from build123d import *

# Parameters (mm, degrees)
CROQUIS1_R              = 1.5
SALIENTE_EXTRUIR1_DEPTH = 1.6
CROQUIS2_W              = 40
CROQUIS2_H              = 3.2
SALIENTE_EXTRUIR2_DEPTH = 40


with BuildPart() as part:
    # Croquis1 → Saliente-Extruir1 (new, symmetric)
    with BuildSketch(Plane.XY):
        with BuildLine():
            Line((-20, -23.5), (20, -23.5))
            Line((20, -23.5), (20, 4.5))
            ThreePointArc((20, 4.5), (14.435028843, 17.935028843), (1, 23.5))
            Line((1, 23.5), (-1, 23.5))
            ThreePointArc((-1, 23.5), (-14.435028843, 17.935028843), (-20, 4.5))
            Line((-20, 4.5), (-20, -23.5))
        make_face()
        with Locations((-15.5, 0)):
            Circle(CROQUIS1_R, mode=Mode.SUBTRACT)
        with Locations((-7.75, 13.423393759)):
            Circle(CROQUIS1_R, mode=Mode.SUBTRACT)
        with Locations((7.75, 13.423393759)):
            Circle(CROQUIS1_R, mode=Mode.SUBTRACT)
        with Locations((15.5, 0)):
            Circle(CROQUIS1_R, mode=Mode.SUBTRACT)
        with Locations((7.75, -13.423393759)):
            Circle(CROQUIS1_R, mode=Mode.SUBTRACT)
        with Locations((-7.75, -13.423393759)):
            Circle(CROQUIS1_R, mode=Mode.SUBTRACT)
        with BuildLine():
            Line((6.5, 7.5), (6.5, -7.5))
            ThreePointArc((6.5, -7.5), (0, -14), (-6.5, -7.5))
            Line((-6.5, -7.5), (-6.5, 7.5))
            ThreePointArc((-6.5, 7.5), (0, 14), (6.5, 7.5))
        make_face(mode=Mode.SUBTRACT)
    extrude(amount=SALIENTE_EXTRUIR1_DEPTH, both=True)

    # Croquis2 → Saliente-Extruir2 (add)
    with BuildSketch(Plane(origin=(0, 0, -1.6), x_dir=(-1, 0, 0), z_dir=(0, 0, -1))):
        with Locations((0, -21.9)):
            Rectangle(CROQUIS2_W, CROQUIS2_H)
    extrude(amount=SALIENTE_EXTRUIR2_DEPTH)


solid = part.part
Source: CAD feature listing. Evaluate the final solid. Frame: model axes, mm. A direction names the side the tool comes from. Coordinates: 2 decimals unless noted, no trailing zeros. Loops run counter-clockwise (first coordinate to the right, second up) from the corner with the lowest first, then second, coordinate; pieces in that order, holes last. Notation, with made-up numbers: (50.5, 65.25) -> (62.5, 65.25) arc R26 cw to (62.5, 92.25) -> close; hole circle Ø2 at (22.5, -22). An arc over 180 degrees is marked (long way). Answer in a Markdown table with one row per item. Add a question column.
Q1. Section D-D on y = -11. Return the cut outline in (x, z).
Q2. Pull-direction query (Y, two-part tool) for faces 4 (the face through (6.5, 0, 0)), 5 (the face through (0, 14, 0)), 6 (the face through (0, -23.5, -20)), 7 (the face through (20, -21, -13)); classes: pulls with the +Y half, pulls with the -Y half, needs draft (parallel to the pull), parting line crosses it, or undercut.
Q3. Section A-A on x = 0. Return the cut outline in (y, z).
Q4. Section B-B on y = -2.5. Return the cut outline in (x, z), and give its area (3 significant figures).
Q5. Contact query for flat-ended pins moving along their axis: pin 1 Ø4 at (x, y) = (7.75, 13.42) entering from -Z; pin 2 Ø12 at (x, z) = (1, -15.5) entering from +Y; pin 3 Ø3 at (x, y) = (5.5, -8.5) entering from +Z; pin 4 Ø12 at (y, z) = (17, -5) entering from +X. Output: stop coordinate, or through.
Q6. Reachability of faces 1 (the face through (-6.5, 0, 0)), 2 (the face through (-20, -21, -13)), 3 (the face through (-9, 2, -1.6)) from +Z, -Z, +X, -X, +Y, -Y: full face, straight path, thin tool, end or side. Return the list, or none.
Q7. Section C-C on x = -7.75. Return the cut outline in (y, z), and give its area (3 significant figures).
Q8. Ray query, line 1 along Z through (x, y) = (11, -18); line 2 along Y through (x, z) = (-10.5, -27); line 3 along Y through (x, z) = (-15, 0). Return the intervals inside material, ascending.
Computed values:
| question | item | result |
|---|---|---|
| 1 | outline | (-20, -1.6) -> (-5.48, -1.6) -> (-5.48, 1.6) -> (-20, 1.6) -> close; (5.48, -1.6) -> (20, -1.6) -> (20, 1.6) -> (5.48, 1.6) -> close |
| 2 | face 4 | undercut |
| 2 | face 5 | undercut |
| 2 | face 6 | pulls with the -Y half |
| 2 | face 7 | needs draft |
| 3 | outline | (-23.5, -41.6) -> (-20.3, -41.6) -> (-20.3, -1.6) -> (-14, -1.6) -> (-14, 1.6) -> (-23.5, 1.6) -> close; (14, -1.6) -> (23.5, -1.6) -> (23.5, 1.6) -> (14, 1.6) -> close |
| 4 | outline | (-20, -1.6) -> (-6.5, -1.6) -> (-6.5, 1.6) -> (-20, 1.6) -> close; (6.5, -1.6) -> (20, -1.6) -> (20, 1.6) -> (6.5, 1.6) -> close |
| 4 | area | 86.4 mm^2 |
| 5 | pin 1 | stops at z = -1.6 |
| 5 | pin 2 | stops at y = -20.3 |
| 5 | pin 3 | stops at z = 1.6 |
| 5 | pin 4 | stops at x = 18.43 |
| 6 | face 1 | +Z, -Z |
| 6 | face 2 | +Z, -Z, -X, +Y, -Y |
| 6 | face 3 | -Z, +X, -X, +Y |
| 7 | outline | (-23.5, -41.6) -> (-20.3, -41.6) -> (-20.3, -1.6) -> (-14.92, -1.6) -> (-14.92, 1.6) -> (-23.5, 1.6) -> close; (-11.92, -1.6) -> (11.92, -1.6) -> (11.92, 1.6) -> (-11.92, 1.6) -> close; (14.92, -1.6) -> (22.26, -1.6) -> (22.26, 1.6) -> (14.92, 1.6) -> close |
| 7 | area | 255 mm^2 |
| 8 | line 1 | z = -1.6 to 1.6 |
| 8 | line 2 | y = -23.5 to -20.3 |
| 8 | line 3 | y = -23.5 to -1.41, 1.41 to 17.35 |
